Verification items for the finished model (mm, model axes). Give positions to 0.01 mm unless a question says otherwise; leave off trailing zeros. Order: outer loops, then holes, each group sorted by start corner. A loop starts at its lowest first (then second) coordinate and runs counter-clockwise, first axis right, second up.
(1) Sectioned sample at C-C on x = 89. Record the cut outline in (y, z), plus the area to 3 significant figures.
(2) Scan lines: L1, parallel to Z at x = -82.5, y = 1.7; L2, parallel to X at y = 1.5, z = 63; L3, parallel to Z at x = 23.5, y = 2.25. Record each from-to range of solid material in increasing order.
(3) Sectioned sample at B-B on y = 1.55. Count the separate pieces of the cut face and the enclosed holes in it, plus the area to 3 significant figures.
(4) Gauge pin test, flat end, axial feed: pin 1 (0.9 mm diameter, centred on x = -118.5, y = 1.5, fed in from +Z). Record the tip position at first contact, or that the pin passes through.
(5) Sectioned sample at A-A on z = -87. Record the cut outline in (x, y), plus the area to 3 significant figures.
```python
from build123d import *

# Parameters (mm, degrees)
SKETCH1_R           = 1.6
SKETCH1_W           = 10.1
SKETCH1_H           = 3.1
SKETCH1_W_2         = 3.1
SKETCH1_H_2         = 10.1
BOSS_EXTRUDE1_DEPTH = 3
CUT_EXTRUDE1_REACH  = 162.106
SKETCH3_R           = 1.35
SKETCH3_R_2         = 1.6
FILLET1_R           = 3


with BuildPart() as part:
    # Sketch1 → Boss-Extrude1 (new body)
    with BuildSketch(Plane(origin=(0, 0, 0), x_dir=(1, 0, 0), z_dir=(0, 1, 0))):
        Polygon((-85, 100), (85, 100), (125, 76.905989232), (125, -76.905989232), (85, -100), (-85, -100), (-125, -76.905989232), (-125, 76.905989232), align=None)
        with Locations(Location((-47.5, -60, 0), (0, 0, 270))):
            Circle(SKETCH1_R, mode=Mode.SUBTRACT)
        with Locations(Location((82.856406461, 92, 0), (0, 0, 270))):
            Circle(SKETCH1_R, mode=Mode.SUBTRACT)
        with Locations(Location((117, 72.287187079, 0), (0, 0, 270))):
            Circle(SKETCH1_R, mode=Mode.SUBTRACT)
        with Locations(Location((117, -72.287187079, 0), (0, 0, 270))):
            Circle(SKETCH1_R, mode=Mode.SUBTRACT)
        with Locations(Location((82.856406461, -92, 0), (0, 0, 270))):
            Circle(SKETCH1_R, mode=Mode.SUBTRACT)
        with Locations(Location((-27.5, -60, 0), (0, 0, 270))):
            Circle(SKETCH1_R, mode=Mode.SUBTRACT)
        with Locations(Location((-27.5, 60, 0), (0, 0, 270))):
            Circle(SKETCH1_R, mode=Mode.SUBTRACT)
        with Locations(Location((-117, -72.287187079, 0), (0, 0, 270))):
            Circle(SKETCH1_R, mode=Mode.SUBTRACT)
        with Locations(Location((-50.5, -92, 0), (0, 0, 270))):
            Circle(SKETCH1_R, mode=Mode.SUBTRACT)
        with Locations(Location((-47.5, 60, 0), (0, 0, 270))):
            Circle(SKETCH1_R, mode=Mode.SUBTRACT)
        with Locations(Location((-117, 72.287187079, 0), (0, 0, 270))):
            Circle(SKETCH1_R, mode=Mode.SUBTRACT)
        with Locations(Location((-50.5, 92, 0), (0, 0, 270))):
            Circle(SKETCH1_R, mode=Mode.SUBTRACT)
        with Locations(Location((-82.856406461, -92, 0), (0, 0, 270))):
            Circle(SKETCH1_R, mode=Mode.SUBTRACT)
        with Locations(Location((-82.856406461, 92, 0), (0, 0, 270))):
            Circle(SKETCH1_R, mode=Mode.SUBTRACT)
        with Locations((-22.45, -93.45)):
            Rectangle(SKETCH1_W, SKETCH1_H, mode=Mode.SUBTRACT)
        with Locations((-118.45, 60)):
            Rectangle(SKETCH1_W_2, SKETCH1_H_2, mode=Mode.SUBTRACT)
        with Locations((-118.45, 20)):
            Rectangle(SKETCH1_W_2, SKETCH1_H_2, mode=Mode.SUBTRACT)
        with Locations((-118.45, -20)):
            Rectangle(SKETCH1_W_2, SKETCH1_H_2, mode=Mode.SUBTRACT)
        with Locations((-118.45, -60)):
            Rectangle(SKETCH1_W_2, SKETCH1_H_2, mode=Mode.SUBTRACT)
        with Locations((118.45, -60)):
            Rectangle(SKETCH1_W_2, SKETCH1_H_2, mode=Mode.SUBTRACT)
        with Locations((118.45, -20)):
            Rectangle(SKETCH1_W_2, SKETCH1_H_2, mode=Mode.SUBTRACT)
        with Locations((118.45, 20)):
            Rectangle(SKETCH1_W_2, SKETCH1_H_2, mode=Mode.SUBTRACT)
        with Locations((118.45, 60)):
            Rectangle(SKETCH1_W_2, SKETCH1_H_2, mode=Mode.SUBTRACT)
        with Locations((22.45, -93.45)):
            Rectangle(SKETCH1_W, SKETCH1_H, mode=Mode.SUBTRACT)
        with Locations((67.35, -93.45)):
            Rectangle(SKETCH1_W, SKETCH1_H, mode=Mode.SUBTRACT)
        with Locations((67.35, 93.45)):
            Rectangle(SKETCH1_W, SKETCH1_H, mode=Mode.SUBTRACT)
        with Locations((22.45, 93.45)):
            Rectangle(SKETCH1_W, SKETCH1_H, mode=Mode.SUBTRACT)
        with Locations((-22.45, 93.45)):
            Rectangle(SKETCH1_W, SKETCH1_H, mode=Mode.SUBTRACT)
    extrude(amount=BOSS_EXTRUDE1_DEPTH)

    # Sketch3 → Cut-Extrude1 (cut, up to next)
    with BuildSketch(Plane(origin=(0, 3, 0), x_dir=(1, 0, 0), z_dir=(0, 1, 0)), mode=Mode.PRIVATE) as cut_extrude1_sk1:
        with Locations(Location((-100, -46, 0), (0, 0, 270))):
            Circle(SKETCH3_R)
    cut_extrude1_tool1 = extrude(cut_extrude1_sk1.sketch, amount=-CUT_EXTRUDE1_REACH, mode=Mode.PRIVATE) & part.part
    # Sketch3 → Cut-Extrude1 (cut, up to next)
    with BuildSketch(Plane(origin=(0, 3, 0), x_dir=(1, 0, 0), z_dir=(0, 1, 0)), mode=Mode.PRIVATE) as cut_extrude1_sk2:
        with Locations(Location((-42, -46, 0), (0, 0, 270))):
            Circle(SKETCH3_R)
    cut_extrude1_tool2 = extrude(cut_extrude1_sk2.sketch, amount=-CUT_EXTRUDE1_REACH, mode=Mode.PRIVATE) & part.part
    # Sketch3 → Cut-Extrude1 (cut, up to next)
    with BuildSketch(Plane(origin=(0, 3, 0), x_dir=(1, 0, 0), z_dir=(0, 1, 0)), mode=Mode.PRIVATE) as cut_extrude1_sk3:
        with Locations(Location((-42, 40, 0), (0, 0, 270))):
            Circle(SKETCH3_R)
    cut_extrude1_tool3 = extrude(cut_extrude1_sk3.sketch, amount=-CUT_EXTRUDE1_REACH, mode=Mode.PRIVATE) & part.part
    # Sketch3 → Cut-Extrude1 (cut, up to next)
    with BuildSketch(Plane(origin=(0, 3, 0), x_dir=(1, 0, 0), z_dir=(0, 1, 0)), mode=Mode.PRIVATE) as cut_extrude1_sk4:
        with Locations(Location((-100, 40, 0), (0, 0, 270))):
            Circle(SKETCH3_R)
    cut_extrude1_tool4 = extrude(cut_extrude1_sk4.sketch, amount=-CUT_EXTRUDE1_REACH, mode=Mode.PRIVATE) & part.part
    # Sketch3 → Cut-Extrude1 (cut, up to next)
    with BuildSketch(Plane(origin=(0, 3, 0), x_dir=(1, 0, 0), z_dir=(0, 1, 0)), mode=Mode.PRIVATE) as cut_extrude1_sk5:
        with Locations(Location((18, 61, 0), (0, 0, 270))):
            Circle(SKETCH3_R_2)
    cut_extrude1_tool5 = extrude(cut_extrude1_sk5.sketch, amount=-CUT_EXTRUDE1_REACH, mode=Mode.PRIVATE) & part.part
    # Sketch3 → Cut-Extrude1 (cut, up to next)
    with BuildSketch(Plane(origin=(0, 3, 0), x_dir=(1, 0, 0), z_dir=(0, 1, 0)), mode=Mode.PRIVATE) as cut_extrude1_sk6:
        with Locations(Location((105, 61, 0), (0, 0, 270))):
            Circle(SKETCH3_R_2)
    cut_extrude1_tool6 = extrude(cut_extrude1_sk6.sketch, amount=-CUT_EXTRUDE1_REACH, mode=Mode.PRIVATE) & part.part
    # Sketch3 → Cut-Extrude1 (cut, up to next)
    with BuildSketch(Plane(origin=(0, 3, 0), x_dir=(1, 0, 0), z_dir=(0, 1, 0)), mode=Mode.PRIVATE) as cut_extrude1_sk7:
        with Locations(Location((105, -61, 0), (0, 0, 270))):
            Circle(SKETCH3_R_2)
    cut_extrude1_tool7 = extrude(cut_extrude1_sk7.sketch, amount=-CUT_EXTRUDE1_REACH, mode=Mode.PRIVATE) & part.part
    # Sketch3 → Cut-Extrude1 (cut, up to next)
    with BuildSketch(Plane(origin=(0, 3, 0), x_dir=(1, 0, 0), z_dir=(0, 1, 0)), mode=Mode.PRIVATE) as cut_extrude1_sk8:
        with Locations(Location((18, -61, 0), (0, 0, 270))):
            Circle(SKETCH3_R_2)
    cut_extrude1_tool8 = extrude(cut_extrude1_sk8.sketch, amount=-CUT_EXTRUDE1_REACH, mode=Mode.PRIVATE) & part.part
    add(cut_extrude1_tool1.solids().sort_by_distance((-100, 3, 46))[0], mode=Mode.SUBTRACT)
    add(cut_extrude1_tool2.solids().sort_by_distance((-42, 3, 46))[0], mode=Mode.SUBTRACT)
    add(cut_extrude1_tool3.solids().sort_by_distance((-42, 3, -40))[0], mode=Mode.SUBTRACT)
    add(cut_extrude1_tool4.solids().sort_by_distance((-100, 3, -40))[0], mode=Mode.SUBTRACT)
    add(cut_extrude1_tool5.solids().sort_by_distance((18, 3, -61))[0], mode=Mode.SUBTRACT)
    add(cut_extrude1_tool6.solids().sort_by_distance((105, 3, -61))[0], mode=Mode.SUBTRACT)
    add(cut_extrude1_tool7.solids().sort_by_distance((105, 3, 61))[0], mode=Mode.SUBTRACT)
    add(cut_extrude1_tool8.solids().sort_by_distance((18, 3, 61))[0], mode=Mode.SUBTRACT)

    # Fillet1
    fillet1_edges = [part.edges().sort_by_distance(p)[0] for p in [
        (-85, 1.5, -100),
        (85, 1.5, -100),
        (125, 1.5, -76.905989232),
        (125, 1.5, 76.905989232),
        (85, 1.5, 100),
        (-85, 1.5, 100),
        (-125, 1.5, 76.905989232),
        (-125, 1.5, -76.905989232),
    ]]
    fillet(fillet1_edges, radius=FILLET1_R)


solid = part.part
```
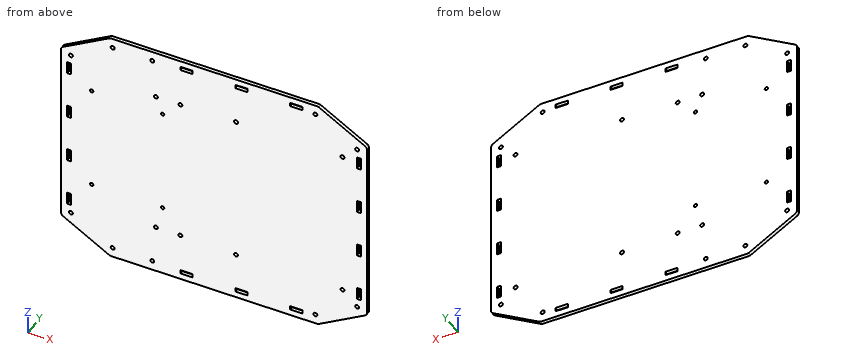
Ans:
1. outline: (0, -97.69) - (3, -97.69) - (3, 97.69) - (0, 97.69) - close
1. area: 586 mm2
2. L1: z = -100 to -93.56, -90.44 to 90.44, 93.56 to 100
2. L2: x = -125 to -120, -116.9 to 116.9, 120 to 125
2. L3: z = -100 to -95, -91.9 to 91.9, 95 to 100
3. separate pieces: 1
3. enclosed holes: 36
3. area: 47,500 mm2
4. pin 1: stops at z = 80.92
5. outline: (-107.52, 0) - (107.52, 0) - (107.52, 3) - (-107.52, 3) - close
5. area: 645 mm2
